Work out the finished part from the listing and answer in its coordinate system (mm). Face numbers are marked on the shaded views. A direction names the side the tool comes from. Give positions to 0.01 mm unless a question says otherwise; leave off trailing zeros. Order: outer loops, then holes, each group sorted by start corner. A loop starts at its lowest first (then second) coordinate and runs counter-clockwise, first axis right, second up.
Autodesk Inventor part; units mm, degrees
ref_plane "YZ Plane" through (0, 0, 0) normal (1, 0, 0) x (0, 1, 0)
ref_plane "XZ Plane" through (0, 0, 0) normal (0, 1, 0) x (-1, 0, 0)
ref_plane "XY Plane" through (0, 0, 0) normal (0, 0, 1) x (1, 0, 0)
sketch "스케치1" plane through (0, 0, 0) normal (0, 1, 0) x (-1, 0, 0)
  line L0 (-12.5, 16) -> (12.5, 16)
  line L1 (12.5, 16) -> (12.5, -16)
  line L2 (12.5, -16) -> (-12.5, -16)
  line L3 (-12.5, -16) -> (-12.5, 16)
  line L4 (-12.5, 16) -> (12.5, -16) construction
  line L5 (12.5, 16) -> (-12.5, -16) construction
  point P0 (0, 0)
  dimension "d0" = 25
  dimension "d1" = 32
extrude "돌출1" add sketch "스케치1" along normal blind 10.16
sketch "스케치4" plane through (0, 0, 0) normal (0, -1, 0) x (1, 0, 0)
  line L0 (-12.5, -16) -> (-12.5, 16)
  line L1 (12.5, 16) -> (12.5, -16)
  line L2 (-12.5, 13.5) -> (12.5, 13.5)
  line L3 (12.5, 13.5) -> (12.5, 8.5)
  line L4 (12.5, 8.5) -> (-12.5, 8.5)
  line L5 (-12.5, 8.5) -> (-12.5, 13.5)
  line L6 (-12.5, 0) -> (12.5, 0)
  line L7 (-12.5, 16) -> (-12.5, -16)
  line L8 (12.5, -10.8) -> (12.5, 10.8)
  line L9 (-12.5, -13.5) -> (12.5, -13.5)
  line L10 (12.5, -13.5) -> (12.5, -8.5)
  line L11 (12.5, -8.5) -> (-12.5, -8.5)
  line L12 (-12.5, -8.5) -> (-12.5, -13.5)
  point P0 (0, 0)
  point P1 (12.5, -8.5)
  point P2 (-12.5, -13.5)
  point P3 (12.5, -13.5)
  point P4 (12.5, 13.5)
  dimension "d13" = 8.5
  dimension "d14" = 5
extrude "돌출4" add sketch "스케치4" along normal blind 10 contours L0 L11 L1 L9 | L0 L2 L1 L4
sketch "스케치5" plane through (12.5, 0, -13.5) normal (0, 0, -1) x (-1, 0, 0)
  circle A0 centre (17.5, -5) radius 1.25
  line L0 (25, -10) -> (0, -10)
  line L1 (25, 0) -> (25, -10)
  line L2 (12.5, -10) -> (12.5, 0)
  circle A1 centre (7.5, -5) radius 1.25
  dimension "d17" = 2.5
  dimension "d18" = 5
  dimension "d22" = 5
extrude "돌출5" cut sketch "스케치5" against normal up to surface (27 mm away)
sketch "스케치6" plane through (0, 10.16, 0) normal (0, 1, 0) x (1, 0, 0)
  circle A0 centre (0, 0) radius 4.5
  line L0 (2.5981, -4.5) -> (-2.5981, -4.5)
  line L1 (-2.5981, -4.5) -> (-5.1962, 0)
  line L2 (-5.1962, 0) -> (-2.5981, 4.5)
  line L3 (-2.5981, 4.5) -> (2.5981, 4.5)
  line L4 (2.5981, 4.5) -> (5.1962, 0)
  line L5 (5.1962, 0) -> (2.5981, -4.5)
  dimension "d25" = 9
extrude "돌출6" cut sketch "스케치6" against normal blind 8
sketch "스케치7" plane through (0, 2.16, 0) normal (0, 1, 0) x (1, 0, 0)
  line L0 (2.5981, 4.5) -> (5.1962, 0)
  line L1 (-2.5981, 4.5) -> (2.5981, 4.5)
  line L2 (-5.1962, 0) -> (-2.5981, 4.5)
  line L3 (-2.5981, -4.5) -> (-5.1962, 0)
  line L4 (2.5981, -4.5) -> (-2.5981, -4.5)
  line L5 (5.1962, 0) -> (2.5981, -4.5)
  line L6 (-2.0207, 3.5) -> (2.0207, 3.5)
  line L7 (2.0207, 3.5) -> (4.0415, 0)
  line L8 (4.0415, 0) -> (2.0207, -3.5)
  line L9 (2.0207, -3.5) -> (-2.0207, -3.5)
  line L10 (-2.0207, -3.5) -> (-4.0415, 0)
  line L11 (-4.0415, 0) -> (-2.0207, 3.5)
  point P0 (0, 0)
  point P1 (0, 0)
  dimension "d29" = 1
extrude "돌출7" add sketch "스케치7" along normal blind 4.5
fillet "모깎기1" radius 0.5 6 edges at (-3.8971, 10.16, 2.25) (0, 10.16, 4.5) (-3.8971, 10.16, -2.25) (0, 10.16, -4.5) (3.8971, 10.16, -2.25) (3.8971, 10.16, 2.25)
properties part number "Tensile_test_bottom_adapter2"
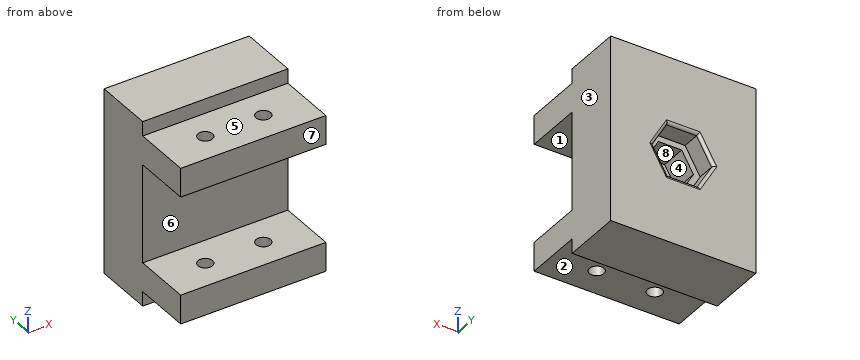
1. Given P1, Ø1.2, axis at x = 2.5, z = 15, coming from the -Y side; P2, Ø5.5, axis at x = -1.5, z = -1.5, coming from the +Y side; P3, Ø5, axis at x = -1, y = -4.5, coming from the +Z side, each flat-ended and moving along its own axis, determine where each tip first touches the part or whether it passes through.
Findings below:
P1: stops at y = 0
P2: stops at y = 10.12
P3: stops at z = 13.5
2. The part is cut by section C-C (z = -12.5). Write down the section's boundary in (x, y), then the cut area to 3 significant figures.
Findings below:
outline: (-12.5, -10) - (12.5, -10) - (12.5, 10.16) - (-12.5, 10.16) - close; hole circle Ø2.5 at (-5, -5); hole circle Ø2.5 at (5, -5)
area: 494 mm2
3. The part is cut by section D-D (y = -5). Write down the section's boundary in (x, z).
Findings below:
outline: (-12.5, -13.5) - (-6.25, -13.5) - (-6.25, -8.5) - (-12.5, -8.5) - close; (-12.5, 8.5) - (-6.25, 8.5) - (-6.25, 13.5) - (-12.5, 13.5) - close; (-3.75, -13.5) - (3.75, -13.5) - (3.75, -8.5) - (-3.75, -8.5) - close; (-3.75, 8.5) - (3.75, 8.5) - (3.75, 13.5) - (-3.75, 13.5) - close; (6.25, -13.5) - (12.5, -13.5) - (12.5, -8.5) - (6.25, -8.5) - close; (6.25, 8.5) - (12.5, 8.5) - (12.5, 13.5) - (6.25, 13.5) - close
4. The part is cut by section B-B (x = -0.5). Write down the section's boundary in (y, z), then the cut area to 3 significant figures.
Findings below:
outline: (-10, -13.5) - (0, -13.5) - (0, -16) - (10.16, -16) - (10.16, -5) arc R0.5 ccw to (9.66, -4.5) - (6.66, -4.5) - (6.66, -3.5) - (2.16, -3.5) - (2.16, 3.5) - (6.66, 3.5) - (6.66, 4.5) - (9.66, 4.5) arc R0.5 ccw to (10.16, 5) - (10.16, 16) - (0, 16) - (0, 13.5) - (-10, 13.5) - (-10, 8.5) - (0, 8.5) - (0, -8.5) - (-10, -8.5) - close
area: 362 mm2
5. Which of the six approach directions +Z, -Z, +X, -X, +Y, -Y give full straight-line access (tool end or side, diameter ignored) to the marked faces 5, 6, 7 and 8?
Findings below:
face 5: +Z, +X, -X, -Y
face 6: +X, -X, -Y
face 7: +Z, -Z, +X, -X, -Y
face 8: +Y
6. Straight lines are drawn through the part: probe 1 along Y at (x, z) = (-5, 11.55); probe 2 along Z at (x, y) = (5, -8.5); probe 3 along Y at (x, z) = (5, 6.5). For each, find the intervals that lie inside material, in ascending order.
Findings below:
probe 1: y = -10 to -6.25, -3.75 to 10.16
probe 2: z = -13.5 to -8.5, 8.5 to 13.5
probe 3: y = 0 to 10.16
7. The part is cut by section A-A (y = -8). Write down the section's boundary in (x, z).
Findings below:
outline: (-12.5, -13.5) - (12.5, -13.5) - (12.5, -8.5) - (-12.5, -8.5) - close; (-12.5, 8.5) - (12.5, 8.5) - (12.5, 13.5) - (-12.5, 13.5) - close
8. The mould has two halves that part along Z. Classify the marked faces 1, 2, 3 and 4: pulls with the +Z half, pulls with the -Z half, needs draft (parallel to the pull), parting line crosses it, or undercut.
Findings below:
face 1: undercut
face 2: pulls with the -Z half
face 3: needs draft
face 4: undercut
